```python
from build123d import *

# Parameters (mm, degrees)
F0_W     = 95
F0_H     = 60
F1_DEPTH = 8
F2_W     = 85.2
F2_H     = 6.1
F3_DEPTH = 25
F4_R     = 1


with BuildPart() as f1:
    # F0 (on Top) → F1 (new body)
    with BuildSketch(Plane.XY):
        with Locations((47.5, 30)):
            Rectangle(F0_W, F0_H)
    extrude(amount=F1_DEPTH)

    # F2 (on face) → F3 (cut)
    with BuildSketch(Plane.XY.offset(8)):
        with Locations((47.5, 51.95)):
            Rectangle(F2_W, F2_H)
        with Locations((47.5, 8.05)):
            Rectangle(F2_W, F2_H)
    extrude(amount=-F3_DEPTH, mode=Mode.SUBTRACT)

    # F4
    f4_edges = [f1.edges().sort_by_distance(p)[0] for p in [
        (0, 60, 4),
        (0, 0, 4),
        (95, 0, 4),
        (95, 60, 4),
        (0, 30, 8),
        (47.5, 0, 8),
        (95, 30, 8),
        (47.5, 60, 8),
    ]]
    fillet(f4_edges, radius=F4_R)


solid = f1.part
```
The model under review builds one solid part; all positions refer to its coordinate system, in mm. A direction names the side the tool comes from. Coordinates: 2 decimals unless noted, no trailing zeros. Order: outer loops, then holes, each group sorted by start corner. A loop starts at its lowest first (then second) coordinate and runs counter-clockwise, first axis right, second up. Notation, with made-up numbers: M 43.25,87 L 85.25,87 A22 ccw 85.25,105 Z; hole C -22.5,-35 d7. An arc over 180 degrees is marked long. One line per question, with ' | ' between items.
(1) The part is to be moulded in two halves that separate along X. For faces 3 (the face through (47, 30, 0)), 4 (the face through (95, 30, 3)), 5 (the face through (47, 5, 4)), say which applies: +X half, -X half, draft (parallel to the pull), parting line (faces both ways), or undercut.
Geometry results:
face 3: draft | face 4: +X half | face 5: undercut
(2) Add section B-B, the plane x = 16.5. Write out the cut boundary in (y, z), then the cut area to 3 significant figures.
Geometry results:
outline: M 0,0 L 5,0 L 5,8 L 1,8 A1 ccw 0,7 Z; M 11.1,0 L 48.9,0 L 48.9,8 L 11.1,8 Z; M 55,0 L 60,0 L 60,7 A1 ccw 59,8 L 55,8 Z | area: 382 mm²
(3) For probe 1 along Y at (x, z) = (9.5, 2); probe 2 along X at (y, z) = (50, 6), list the stretches that pass through material, from the lowest coordinate up. Write a range as from..to.
Geometry results:
probe 1: y = 0..5, 11.1..48.9, 55..60 | probe 2: x = 0..4.9, 90.1..95
(4) Machinability: for faces 1 (the face through (4.9, 52, 4)), 2 (the face through (0, 30, 3)), which of the approach directions +Z, -Z, +X, -X, +Y, -Y give a long, thin tool a straight path to every point of the face, cutting with its end or side? Answer none if there is none.
Geometry results:
face 1: +Z, -Z | face 2: +Z, -Z, -X, +Y, -Y
(5) Add section A-A, the plane y = 51.5. Write out the cut boundary in (x, z).
Geometry results:
outline: M 0,0 L 4.9,0 L 4.9,8 L 1,8 A1 ccw 0,7 Z; M 90.1,0 L 95,0 L 95,7 A1 ccw 94,8 L 90.1,8 Z
(6) Add section C-C, the plane z = 4.5. Write out the cut boundary in (x, y), then the cut area to 3 significant figures.
Geometry results:
outline: M 0,1 A1 ccw 1,0 L 94,0 A1 ccw 95,1 L 95,59 A1 ccw 94,60 L 1,60 A1 ccw 0,59 Z; hole M 4.9,5 L 90.1,5 L 90.1,11.1 L 4.9,11.1 Z; hole M 4.9,48.9 L 90.1,48.9 L 90.1,55 L 4.9,55 Z | area: 4,660 mm²
